Design review of the part built by this model. Coordinates are the model's own, in mm. Face numbers are marked on the shaded views. A direction names the side the tool comes from. Give positions to 0.01 mm unless a question says otherwise; leave off trailing zeros. Order: outer loops, then holes, each group sorted by start corner. A loop starts at its lowest first (then second) coordinate and runs counter-clockwise, first axis right, second up. Notation, with made-up numbers: (41.5, -13) -> (48.5, -13) arc R30 ccw to (48.5, 24) -> close; hole circle Ø3 at (41, 8). An arc over 180 degrees is marked (long way). Return JSON: item names as keys, results as strings.
```python
from build123d import *

# Parameters (mm, degrees)
SKETCH1_W               = 91
SKETCH1_H               = 12.5
SKETCH2_W               = 31.25
SKETCH2_H               = 62.5
CUT_EXTRUDE1_DEPTH      = 25
CUT_EXTRUDE1_DEPTH_BACK = 25


with BuildPart() as part:
    # Sketch1 → Revolve1 (revolve)
    with BuildSketch(Plane.XY):
        with Locations((34.5, 6.25)):
            Rectangle(SKETCH1_W, SKETCH1_H)
    revolve(axis=Axis((80, 0, 0), (-1, 0, 0)))

    # Sketch2 → Revolve2 (revolve)
    with BuildSketch(Plane.XY):
        with Locations((64.375, 31.25)):
            Rectangle(SKETCH2_W, SKETCH2_H)
    revolve(axis=Axis((80, 0, 0), (-1, 0, 0)))

    # Sketch3 → Cut-Extrude1 (cut, two sides)
    with BuildSketch(Plane.XY) as cut_extrude1_sk:
        Polygon((-67, -28), (8.103629711, -28), (-2, -10.5), (-11, -10.5), (-11, -15.5), (-56, -15.5), (-56, 15.5), (-11, 15.5), (-11, 10.5), (-2, 10.5), (8.103629711, 28), (-67, 28), align=None)
    extrude(amount=CUT_EXTRUDE1_DEPTH, mode=Mode.SUBTRACT)
    extrude(cut_extrude1_sk.sketch, amount=-CUT_EXTRUDE1_DEPTH_BACK, mode=Mode.SUBTRACT)

    # Sketch4 → Cut-Revolve1 (revolve, cut)
    with BuildSketch(Plane.XY):
        Polygon((-11, 0), (-11, 9.5), (-10, 8.5), (-4, 8.5), (-4, 8), (-2.9175, 6.9175), (20.5, 6.9175), (24.493820487, 0), align=None)
    revolve(axis=Axis((24.493820487, 0, 0), (-1, 0, 0)), mode=Mode.SUBTRACT)


solid = part.part
```
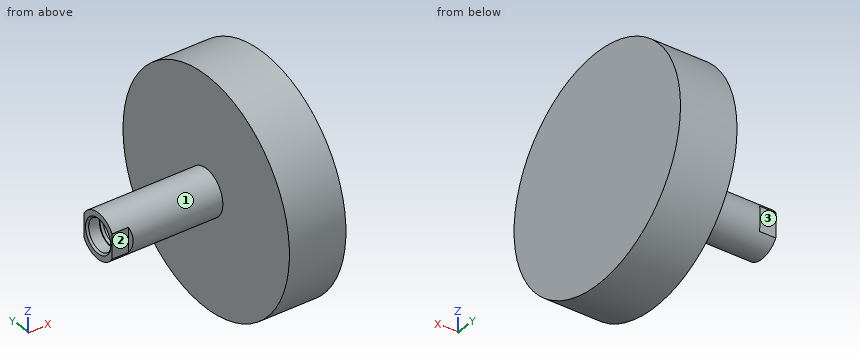
Item 1: For pin 1 (2.5 mm diameter, centred on x = -7.5, z = -3, fed in from -Y); pin 2 (6 mm diameter, centred on y = -44.5, z = 39, fed in from -X); pin 3 (4 mm diameter, centred on x = 50.5, z = -35.5, fed in from +Y); pin 4 (6 mm diameter, centred on x = 43.5, y = 38.5, fed in from -Z), all flat-tipped, find the tip position at first contact; note any pin that passes through.
Result set:
{"pin 1": "stops at y = -10.5", "pin 2": "stops at x = 48.75", "pin 3": "stops at y = 52.76", "pin 4": "passes through"}
Item 2: Add section B-B (z = 26). Give the boundary of the cut face in (x, y), plus the area to 3 significant figures.
Result set:
{"outline": "(48.75, -56.84) -> (80, -56.84) -> (80, 56.84) -> (48.75, 56.84) -> close", "area": "3,550 mm^2"}
Item 3: Machinability: for the marked faces 1, 2 and 3, which of the approach directions +Z, -Z, +X, -X, +Y, -Y give a long, thin tool a straight path to every point of the face, cutting with its end or side? Answer none if there is none.
Result set:
{"face 1": "-X", "face 2": "+Z, -Z, -X, -Y", "face 3": "+Z, -Z, -X, +Y"}
Item 4: Add section C-C (y = 17). Give the boundary of the cut face in (x, z), plus the area to 3 significant figures.
Result set:
{"outline": "(48.75, -60.14) -> (80, -60.14) -> (80, 60.14) -> (48.75, 60.14) -> close", "area": "3,760 mm^2"}
Item 5: Wall thickness on L1, parallel to Z at x = 10.5, y = 0; L2, parallel to Z at x = -6, y = 0: over which ranges is each line inside the solid? List them lowest first. Write a range as [from, to].
Result set:
{"L1": "z = [-12.5, -6.92], [6.92, 12.5]", "L2": "z = [-12.5, -8.5], [8.5, 12.5]"}
Item 6: Add section A-A (x = 55). Give the boundary of the cut face in (y, z).
Result set:
{"outline": "circle Ø125 at (0, 0)"}
